For this review, use the dimensioned drawing (mm, ordinates from the lowest corner) and the shaded views. A direction names the side the tool comes from. Give positions to 0.01 mm unless a question says otherwise; leave off trailing zeros. Write each loop counter-clockwise with the first axis right and the second up, starting at its lowest first coordinate (ties: lowest second). Pieces come first, ordered by that corner, then holes. Notation, with made-up numbers: (82, 20) -> (97, 20) arc R6 cw to (97, 26) -> close; hole circle Ø4 at (35.25, -35). An arc over 180 degrees is marked (long way). Return JSON: item names as keys, results as strings.
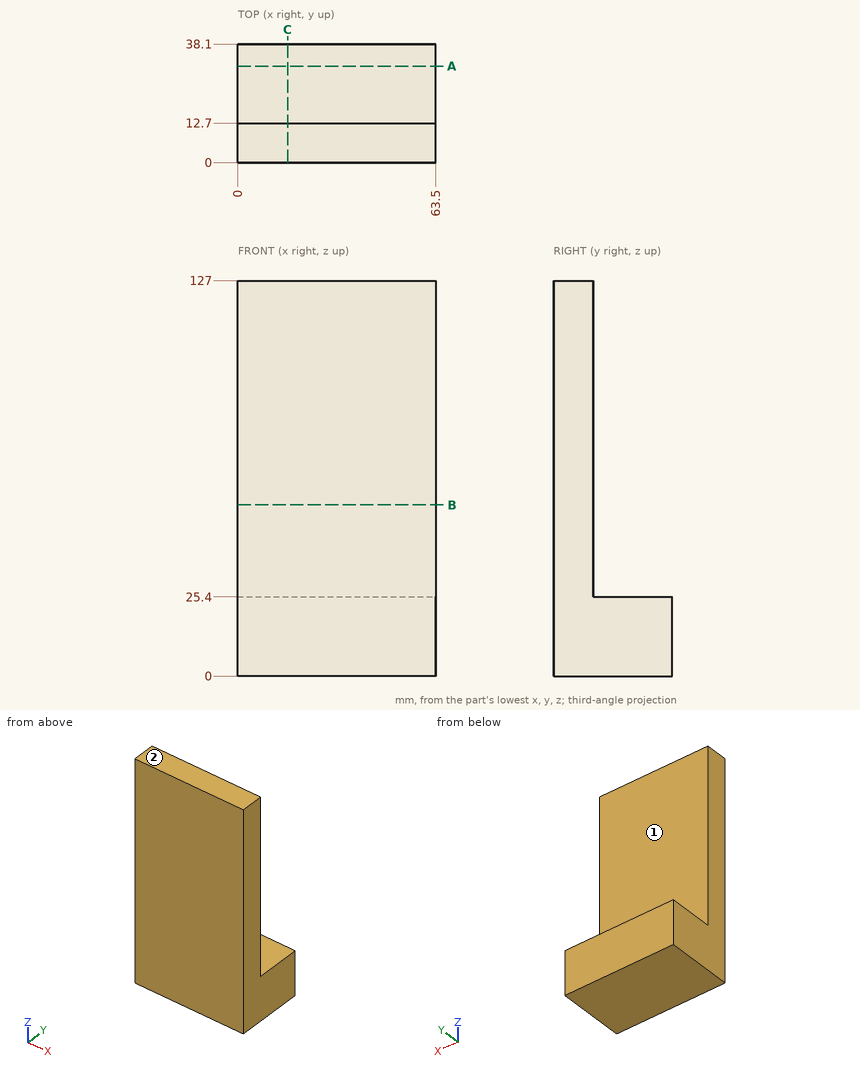
1. For the marked faces 1 and 2, list the 3-axis set-ups (+Z, -Z, +X, -X, +Y, -Y) from which the entire face can be reached by the end or side of a thin tool; tool diameter is ignored.
Results found:
{"face 1": "+Z, +X, -X, +Y", "face 2": "+Z, +X, -X, +Y, -Y"}
2. For pin 1 (3 mm diameter, centred on y = 14.5, z = 79.5, fed in from +X); pin 2 (5 mm diameter, centred on x = 30, y = 24.5, fed in from +Z); pin 3 (1 mm diameter, centred on x = 28.5, z = 82, fed in from +Y), all flat-tipped, find the tip position at first contact; note any pin that passes through.
Results found:
{"pin 1": "passes through", "pin 2": "stops at z = 25.4", "pin 3": "stops at y = 12.7"}
3. Add section B-B, the plane z = 55. State the section outline as (x, y) points, plus the area to 3 significant figures.
Results found:
{"outline": "(0, 0) -> (63.5, 0) -> (63.5, 12.7) -> (0, 12.7) -> close", "area": "806 mm²"}
4. Add section C-C, the plane x = 16. State the section outline as (y, z) points, plus the area to 3 significant figures.
Results found:
{"outline": "(0, 0) -> (38.1, 0) -> (38.1, 25.4) -> (12.7, 25.4) -> (12.7, 127) -> (0, 127) -> close", "area": "2,260 mm²"}
5. Add section A-A, the plane y = 31. State the section outline as (x, z) points, plus the area to 3 significant figures.
Results found:
{"outline": "(0, 0) -> (63.5, 0) -> (63.5, 25.4) -> (0, 25.4) -> close", "area": "1,610 mm²"}
6. To check wall thickness, follow probe 1 along Z at (x, y) = (54.5, 29); probe 2 along Y at (x, z) = (33, 42). State the ranges of each line that lie inside material, in increasing order.
Results found:
{"probe 1": "z = 0 to 25.4", "probe 2": "y = 0 to 12.7"}
